Here's how the part is built. I have some questions about the finished solid (model axes, mm). Face numbers are marked on the shaded views. A direction names the side the tool comes from. Round coordinates to 2 decimals unless told otherwise and drop trailing zeros. Write each loop counter-clockwise with the first axis right and the second up, starting at its lowest first coordinate (ties: lowest second). Pieces come first, ordered by that corner, then holes. Notation, with made-up numbers: M 84.25,-32 L 120.25,-32 A33 cw 120.25,1 Z; hole C 5.25,27.25 d8. An arc over 180 degrees is marked long. Use one line per item in the form item = value. Start each with the question number.
Q1. I want a section at B-B on z = 34.5. List the corners of the cut face in (x, y) for me, and give its area (3 significant figures).
Q2. We'd pull the mould along Y, two halves only. Please class the marked faces 1, 2 and 3: +Y half, -Y half, draft (parallel to the pull), parting line (faces both ways), or undercut.
Q3. I want a section at C-C on x = 2.25. List the corners of the cut face in (y, z) for me.
Q4. I want a section at A-A on y = 0. List the corners of the cut face in (x, z) for me, and give its area (3 significant figures).
Q5. I'm going to push flat-ended pins straight in: pin 1 Ø4.5 at (x, y) = (0.5, 0.5) entering from -Z; pin 2 Ø5 at (x, z) = (-3, 27) entering from +Y; pin 3 Ø1 at (x, z) = (2.5, 6) entering from -Y. Where does each tip first touch, or does it pass through?
Q6. For the marked faces 4 and 5, which set-ups out of +Z, -Z, +X, -X, +Y, -Y let a thin tool reach every point of the face, with its end or its side?
Q7. I need wall thicknesses on line 1 along X through (y, z) = (-2.5, 4); line 2 along Z through (x, y) = (-4.25, 0); line 3 along Z through (x, y) = (-6, 0.25). Which ranges of each line are inside material? Lowest first, please. Write a range as from..to.
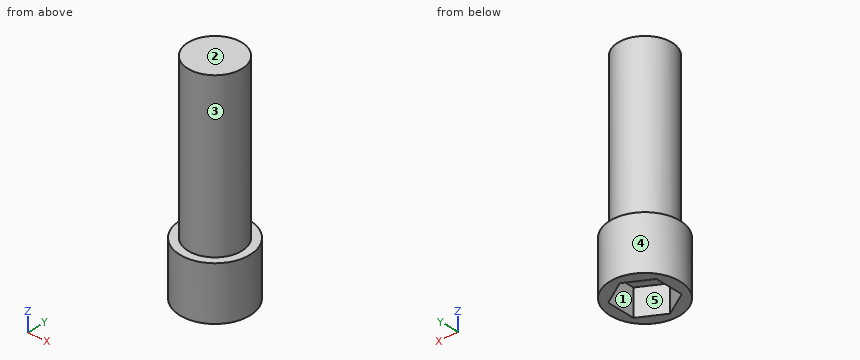
```python
from build123d import *

# Parameters (mm, degrees)
SKETCH1_R           = 6.5
BOSS_EXTRUDE1_DEPTH = 10
SKETCH2_R           = 5
BOSS_EXTRUDE2_DEPTH = 30
CUT_EXTRUDE1_DEPTH  = 5


with BuildPart() as part:
    # Sketch1 → Boss-Extrude1 (new body)
    with BuildSketch(Plane.XY):
        Circle(SKETCH1_R)
    extrude(amount=BOSS_EXTRUDE1_DEPTH)

    # Sketch2 → Boss-Extrude2 (add)
    with BuildSketch(Plane.XY.offset(10)):
        Circle(SKETCH2_R)
    extrude(amount=BOSS_EXTRUDE2_DEPTH)

    # Sketch3 → Cut-Extrude1 (cut)
    with BuildSketch(Plane(origin=(0, 0, 0), x_dir=(-1, 0, 0), z_dir=(0, 0, -1))):
        Polygon((4.5, 2.598076211), (0, 5.196152423), (-4.5, 2.598076211), (-4.5, -2.598076211), (0, -5.196152423), (4.5, -2.598076211), align=None)
    extrude(amount=-CUT_EXTRUDE1_DEPTH, mode=Mode.SUBTRACT)


solid = part.part
```
Reported:
q1.outline = C 0,0 d10
q1.area = 78.5 mm^2
q2.face_1 = undercut
q2.face_2 = draft
q2.face_3 = parting line
q3.outline = M -6.1,0 L -3.9,0 L -3.9,5 L 3.9,5 L 3.9,0 L 6.1,0 L 6.1,10 L 4.47,10 L 4.47,40 L -4.47,40 L -4.47,10 L -6.1,10 Z
q4.outline = M -6.5,0 L -4.5,0 L -4.5,5 L 4.5,5 L 4.5,0 L 6.5,0 L 6.5,10 L 5,10 L 5,40 L -5,40 L -5,10 L -6.5,10 Z
q4.area = 385 mm^2
q5.pin_1 = 5
q5.pin_2 = 4.97
q5.pin_3 = -6.18
q6.face_4 = +Z, -Z
q6.face_5 = -Z
q7.line_1 = -6..-4.5, 4.5..6
q7.line_2 = 5..40
q7.line_3 = 0..10
